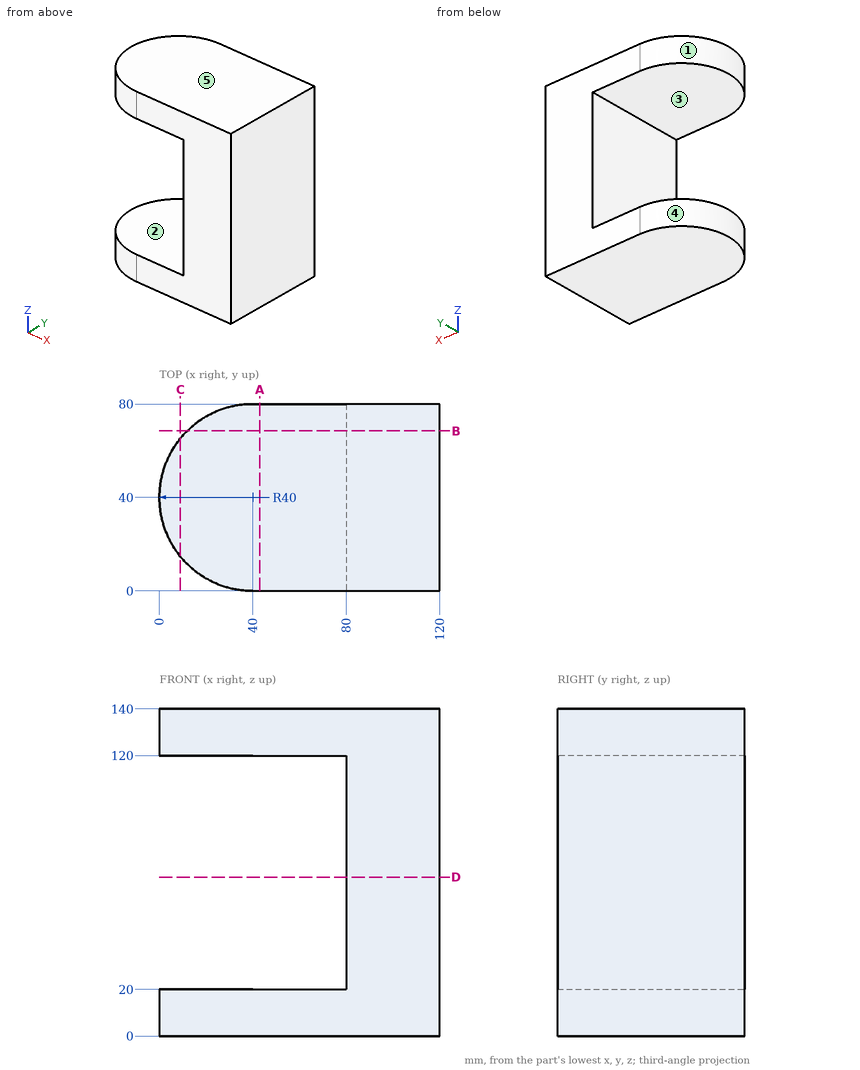
For this review, use the dimensioned drawing (mm, ordinates from the lowest corner) and the shaded views. A direction names the side the tool comes from. Give positions to 0.01 mm unless a question says otherwise; leave off trailing zeros. Write each loop counter-clockwise with the first axis right and the second up, starting at its lowest first coordinate (ties: lowest second). Pieces come first, ordered by that corner, then holes.
(1) Consider section A-A, the plane x = 43. Give the boundary of the cut face in (y, z), and give its area (3 significant figures).
(2) To check wall thickness, follow L1, parallel to Z at x = 49.5, y = 34.5; L2, parallel to X at y = 67.5, z = 58.5; L3, parallel to Y at x = 10, z = 125.5. State the ranges of each line that lie inside material, in increasing order.
(3) Consider section C-C, the plane x = 9. Give the boundary of the cut face in (y, z).
(4) For P1, Ø1.5, axis at y = 39, z = 37.5, coming from the -X side, flat-tipped, find the tip position at first contact; note if it passes through.
(5) Consider section D-D, the plane z = 68. Give the boundary of the cut face in (x, y), and give its area (3 significant figures).
(6) Tool access review of the marked faces 1 and 2: name each direction out of +Z, -Z, +X, -X, +Y, -Y from which nothing blocks a thin tool from reaching the whole face with its end or side.
(7) Consider section B-B, the plane y = 68.5. Give the boundary of the cut face in (x, z), and give its area (3 significant figures).
(8) The part is to be moulded in two halves that separate along Z. For the marked faces 3, 4 and 5, say which applies: released by +Z, released by -Z, zero draft, split by the parting line, or undercut.
Returned:
1. outline: (0, 0) - (80, 0) - (80, 20) - (0, 20) - close; (0, 120) - (80, 120) - (80, 140) - (0, 140) - close
1. area: 3,200 mm2
2. L1: z = 0 to 20, 120 to 140
2. L2: x = 80 to 120
2. L3: y = 13.54 to 66.46
3. outline: (14.72, 0) - (65.28, 0) - (65.28, 20) - (14.72, 20) - close; (14.72, 120) - (65.28, 120) - (65.28, 140) - (14.72, 140) - close
4. P1: stops at x = 80
5. outline: (80, 0) - (120, 0) - (120, 80) - (80, 80) - close
5. area: 3,200 mm2
6. face 1: +Z, -Z, -X
6. face 2: -X, +Y, -Y
7. outline: (11.93, 0) - (120, 0) - (120, 140) - (11.93, 140) - (11.93, 120) - (80, 120) - (80, 20) - (11.93, 20) - close
7. area: 8,320 mm2
8. face 3: undercut
8. face 4: zero draft
8. face 5: released by +Z
